Can you work these out from the model? Positions are in its coordinate system, mm. Face numbers are marked on the shaded views. A direction names the side the tool comes from. Coordinates: 2 decimals unless noted, no trailing zeros. Loops run counter-clockwise (first coordinate to the right, second up) from the corner with the lowest first, then second, coordinate; pieces in that order, holes last.
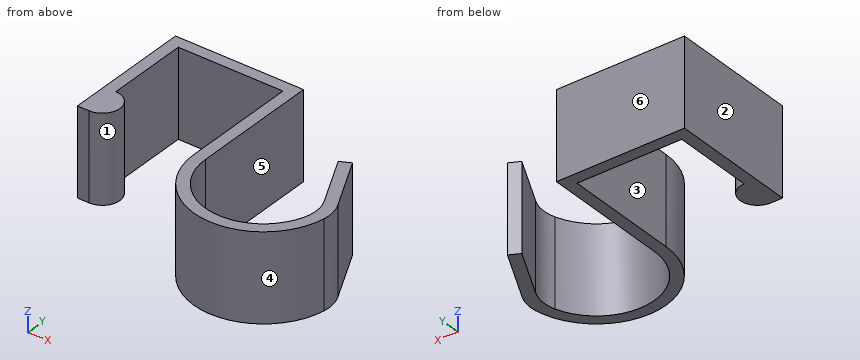
```python
from build123d import *

# Parameters (mm, degrees)
F1_DEPTH = 15


with BuildPart() as f1:
    # F0 (on Top) → F1 (new body)
    with BuildSketch(Plane.XY):
        with BuildLine():
            Line((0, 22), (0, 0))
            Line((0, 0), (2, 0))
            ThreePointArc((2, 0), (5, 3), (2, 6))
            Line((2, 6), (2, 20))
            Line((2, 20), (20, 20))
            Line((20, 20), (20, 0))
            ThreePointArc((20, 0), (31.051796, -11.962479), (43.850152, -1.890478))
            ThreePointArc((43.850152, -1.890478), (43.854746, 0.081043), (43.254428, 1.958949))
            Line((43.254428, 1.958949), (38.442937, 11.542894))
            Line((38.442937, 11.542894), (36.655541, 10.645556))
            Line((36.655541, 10.645556), (41.142232, 1.708576))
            ThreePointArc((41.142232, 1.708576), (41.79999, -0.672597), (41.499315, -3.124582))
            ThreePointArc((41.499315, -3.124582), (30.417779, -9.874035), (22, 0))
            Line((22, 0), (22, 22))
            Line((22, 22), (0, 22))
        make_face()
    extrude(amount=F1_DEPTH)


solid = f1.part
```
Item 1: I need wall thicknesses on line 1 along X through (y, z) = (15, 2.75); line 2 along X through (y, z) = (1, 5.5); line 3 along X through (y, z) = (2, 7.5). Which ranges of each line are inside material? Lowest first, please.
Results are:
line 1: x = 0 to 2, 20 to 22
line 2: x = 0 to 4.24, 20 to 22, 41.45 to 43.64
line 3: x = 0 to 4.83, 20 to 22, 41 to 43.23
Item 2: On a 3-axis mill with a long thin cutter (end or side, diameter ignored), from which of +Z, -Z, +X, -X, +Y, -Y can I reach the whole of each face in a straight line? I mean the marked faces 1 and 2. Say none if no direction works.
Results are:
face 1: +Z, -Z
face 2: +Z, -Z, -X, +Y, -Y
Item 3: I'm going to push flat-ended pins straight in: P1, Ø5, axis at x = 23.5, z = 9, coming from the +Y side; P2, Ø1.5, axis at x = 32.5, z = 7.5, coming from the +Y side; P3, Ø2, axis at y = -7, z = 12.5, coming from the +X side; P4, Ø7, axis at y = 13.5, z = 5.5, coming from the +X side. Where does each tip first touch, or does it pass through?
Results are:
P1: stops at y = 22
P2: stops at y = -9.92
P3: stops at x = 42.39
P4: stops at x = 39.22
Item 4: Suppose I cut it at A-A, the plane y = 16.5. Please give me the cut outline in (x, z).
Results are:
outline: (0, 0) - (2, 0) - (2, 15) - (0, 15) - close; (20, 0) - (22, 0) - (22, 15) - (20, 15) - close
Item 5: We'd pull the mould along X, two halves only. Please class the marked faces 3, 4, 5 and 6: +X half, -X half, draft (parallel to the pull), parting line (faces both ways), or undercut.
Results are:
face 3: undercut
face 4: parting line
face 5: undercut
face 6: draft
Item 6: Suppose I cut it at B-B, the plane z = 8.75. Please give me the cut outline in (x, y), plus the area to 3 significant figures.
Results are:
outline: (0, 0) - (2, 0) arc R3 ccw to (2, 6) - (2, 20) - (20, 20) - (20, 0) arc R12 ccw to (43.85, -1.89) arc R6.35 ccw to (43.25, 1.96) - (38.44, 11.54) - (36.66, 10.65) - (41.14, 1.71) arc R6.35 cw to (41.5, -3.12) arc R10 cw to (22, 0) - (22, 22) - (0, 22) - close
area: 232 mm2
Item 7: Suppose I cut it at C-C, the plane y = 3. Please give me the cut outline in (x, z), plus the area to 3 significant figures.
Results are:
outline: (0, 0) - (5, 0) - (5, 15) - (0, 15) - close; (20, 0) - (22, 0) - (22, 15) - (20, 15) - close; (40.49, 0) - (42.73, 0) - (42.73, 15) - (40.49, 15) - close
area: 139 mm2
Item 8: Suppose I cut it at D-D, the plane x = 9.5. Please give me the cut outline in (y, z), plus the area to 3 significant figures.
Results are:
outline: (20, 0) - (22, 0) - (22, 15) - (20, 15) - close
area: 30.0 mm2
